```python
from build123d import *

# Parameters (mm, degrees)
SKETCH_1_W              = 29.177684157
SKETCH_1_H              = 20
EXTRUDE_1_DEPTH         = 3
SKETCH2_R               = 2
BOSS_EXTRUDE3_DEPTH     = 3
SKETCH_2_R              = 2.5
SKETCH_2_R_2            = 1
CUT_EXTRUDE1_DEPTH      = 10
CUT_EXTRUDE1_DEPTH_BACK = 6


with BuildPart() as part:
    # 草圖1 → 填料-伸長1 (new body)
    with BuildSketch(Plane.XY):
        with Locations((8.493155936, 3.641078838)):
            Rectangle(SKETCH_1_W, SKETCH_1_H)
    extrude(amount=EXTRUDE_1_DEPTH)

    # Sketch2 → Boss-Extrude3 (add)
    with BuildSketch(Plane.XY):
        with Locations((15.993155937, 3.641078838)):
            Circle(SKETCH2_R)
        with Locations((0.993155937, 3.641078838)):
            Circle(SKETCH2_R)
    extrude(amount=-BOSS_EXTRUDE3_DEPTH)

    # 草圖2 → Cut-Extrude1 (cut, two sides)
    with BuildSketch(Plane.XY) as cut_extrude1_sk:
        with Locations((8.493155937, 3.641078838)):
            Circle(SKETCH_2_R)
        with Locations((15.993155937, 3.641078838)):
            Circle(SKETCH_2_R_2)
        with Locations((0.993155937, 3.641078838)):
            Circle(SKETCH_2_R_2)
    extrude(amount=CUT_EXTRUDE1_DEPTH, mode=Mode.SUBTRACT)
    extrude(cut_extrude1_sk.sketch, amount=-CUT_EXTRUDE1_DEPTH_BACK, mode=Mode.SUBTRACT)


solid = part.part
```
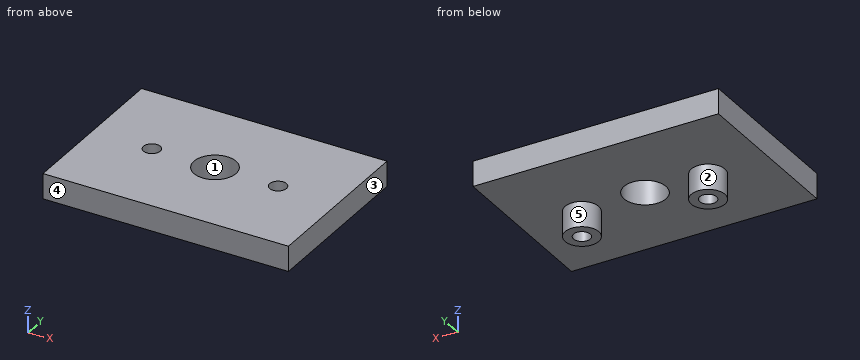
The model under review builds one solid part; all positions refer to its coordinate system, in mm. Face numbers are marked on the shaded views. A direction names the side the tool comes from. Give positions to 0.01 mm unless a question says otherwise; leave off trailing zeros. Write each loop counter-clockwise with the first axis right and the second up, starting at its lowest first coordinate (ties: lowest second). Pieces come first, ordered by that corner, then holes. Notation, with made-up numbers: M 76.5,14.5 L 110.5,14.5 A17 ccw 110.5,26.5 Z; hole C -30.75,88 d11. An arc over 180 degrees is marked long. Write each question's results on one line, items separated by ' | '. Start each with the question number.
1. For the marked faces 4 and 5, list the 3-axis set-ups (+Z, -Z, +X, -X, +Y, -Y) from which the entire face can be reached by the end or side of a thin tool; tool diameter is ignored.
2. We need section B-B (x = 17.5). Write out the cut boundary in (y, z).
3. We need section D-D (z = -2). Write out the cut boundary in (x, y), and give its area (3 significant figures).
4. Insertion check: pin 1 Ø2 at (x, y) = (-3, 8) entering from -Z; pin 2 Ø2 at (y, z) = (-4.5, -2.5) entering from -X. Each pin has a flat end and moves straight along its axis. Give the tip position at first contact, or say it passes through.
5. We need section C-C (y = 8). Write out the cut boundary in (x, z), and give its area (3 significant figures).
6. Mouldability with a two-part tool opening along Y and no side actions: class the marked faces 1, 2 and 3 as released by +Y, released by -Y, zero draft, split by the parting line, or undercut.
7. We need section A-A (z = 2.55). Write out the cut boundary in (x, y).
8. For probe 1 along Y at (x, z) = (10, 1.75); probe 2 along X at (y, z) = (3.5, 0.3); probe 3 along Z at (x, y) = (11.25, -1.75), list the stretches that pass through material, from the lowest coordinate up. Write a range as [from, to].
Results found:
1) face 4: +Z, -Z, +X, -X, -Y | face 5: -Z
2) outline: M -6.36,0 L 2.33,0 L 2.33,-3 L 4.96,-3 L 4.96,0 L 13.64,0 L 13.64,3 L -6.36,3 Z
3) outline: C 0.99,3.64 d4; C 15.99,3.64 d4; hole C 0.99,3.64 d2; hole C 15.99,3.64 d2 | area: 18.8 mm^2
4) pin 1: stops at z = 0 | pin 2: passes through
5) outline: M -6.1,0 L 23.08,0 L 23.08,3 L -6.1,3 Z | area: 87.5 mm^2
6) face 1: undercut | face 2: split by the parting line | face 3: zero draft
7) outline: M -6.1,-6.36 L 23.08,-6.36 L 23.08,13.64 L -6.1,13.64 Z; hole C 0.99,3.64 d2; hole C 8.49,3.64 d5; hole C 15.99,3.64 d2
8) probe 1: y = [-6.36, 1.65], [5.64, 13.64] | probe 2: x = [-6.1, 0], [1.98, 6], [10.99, 15], [16.98, 23.08] | probe 3: z = [0, 3]
